Can you work these out from the model? Positions are in its coordinate system, mm. A direction names the side the tool comes from. Coordinates: 2 decimals unless noted, no trailing zeros. Order: outer loops, then holes, each group sorted by start corner. A loop starts at its lowest first (then second) coordinate and runs counter-clockwise, first axis right, second up. Notation, with made-up numbers: (27, 44) -> (77, 44) arc R9 ccw to (77, 49) -> close; hole circle Ø5 at (-36, -11.5). An arc over 180 degrees is marked (long way). Answer as a JSON object with one key per item and string values. Group by question number.
(1) I want a section at B-B, the plane z = 0. List the corners of the cut face in (x, y) for me.
(2) I need wall thicknesses on line 1 (Y direction, x = 1.5, z = -1.75); line 2 (Y direction, x = 1.5, z = 2.75); line 3 (X direction, y = 4.5, z = 0). Which ranges of each line are inside material? Lowest first, please.
(3) Which directions (+Z, -Z, +X, -X, +Y, -Y) give clear straight access to the entire face, cutting with the end or side of a thin tool? Please do faces 4 (the flat face through (0, 0, 0)), 5 (the cylindrical face through (2.024, 23.493, 1.29)), 6 (the flat face through (-2, 22, -1)).
(4) I want a section at D-D, the plane z = 3. List the corners of the cut face in (x, y) for me.
(5) I want a section at A-A, the plane x = 0. List the corners of the cut face in (y, z) for me, plus the area to 3 significant figures.
(6) If we mould it in two halves opening along Y, with no side actions, what happens to faces 1 (the cylindrical face through (-1, 22.49, -1.31)), 2 (the flat face through (0, 24, 0)), 3 (the cylindrical face through (-3.417, 0.493, -0.759))? For each: pulls with the +Y half, pulls with the -Y half, needs draft (parallel to the pull), parting line crosses it, or undercut.
(7) For pin 1 (3 mm diameter, centred on x = 1.5, y = 9, fed in from -Z); pin 2 (2 mm diameter, centred on y = 5.5, z = -3, fed in from +X); pin 3 (1 mm diameter, centred on y = 4.5, z = -2, fed in from +X), each with a flat end and sliding along its axis, tell me the tip position at first contact or that it passes through.
(8) I want a section at C-C, the plane y = 19.75. List the corners of the cut face in (x, z) for me.
from build123d import *

# Parameters (mm, degrees)
CROQUIS1_R              = 3.5
CROQUIS1_R_2            = 2.4
SALIENTE_EXTRUIR1_DEPTH = 1
CROQUIS1_2_R            = 2.4
SALIENTE_EXTRUIR2_DEPTH = 24
CORTAR_EXTRUIR1_START   = -2
CROQUIS2_R              = 2.4
CROQUIS2_R_2            = 1.65
CORTAR_EXTRUIR1_DEPTH   = 1


with BuildPart() as part:
    # Croquis1 → Saliente-Extruir1 (new body)
    with BuildSketch(Plane(origin=(0, 0, 0), x_dir=(1, 0, 0), z_dir=(0, 1, 0))):
        with Locations(Location((0, 0, 0), (0, 0, 270))):
            Circle(CROQUIS1_R)
        with Locations(Location((0, 0, 0), (0, 0, 270))):
            Circle(CROQUIS1_R_2, mode=Mode.SUBTRACT)
    extrude(amount=SALIENTE_EXTRUIR1_DEPTH)

    # Croquis1_2 → Saliente-Extruir2 (add)
    with BuildSketch(Plane(origin=(0, 0, 0), x_dir=(1, 0, 0), z_dir=(0, 1, 0))):
        with Locations(Location((0, 0, 0), (0, 0, 270))):
            Circle(CROQUIS1_2_R)
    extrude(amount=SALIENTE_EXTRUIR2_DEPTH)

    # Croquis2 → Cortar-Extruir1 (cut)
    with BuildSketch(Plane(origin=(0, 24, 0), x_dir=(1, 0, 0), z_dir=(0, 1, 0)).offset(CORTAR_EXTRUIR1_START)):
        with Locations(Location((0, 0, 0), (0, 0, 270))):
            Circle(CROQUIS2_R)
        with Locations(Location((0, 0, 0), (0, 0, 270))):
            Circle(CROQUIS2_R_2, mode=Mode.SUBTRACT)
    extrude(amount=CORTAR_EXTRUIR1_DEPTH, mode=Mode.SUBTRACT)


solid = part.part
Computed values:
{
 "1": {"outline": "(-3.5, 0) -> (3.5, 0) -> (3.5, 1) -> (2.4, 1) -> (2.4, 22) -> (1.65, 22) -> (1.65, 23) -> (2.4, 23) -> (2.4, 24) -> (-2.4, 24) -> (-2.4, 23) -> (-1.65, 23) -> (-1.65, 22) -> (-2.4, 22) -> (-2.4, 1) -> (-3.5, 1) -> close"},
 "2": {"line 1": "y = 0 to 22, 23 to 24", "line 2": "y = 0 to 1", "line 3": "x = -2.4 to 2.4"},
 "3": {"face 4": "+Z, -Z, +X, -X, -Y", "face 5": "+Y", "face 6": "none"},
 "4": {"outline": "(-1.8, 0) -> (1.8, 0) -> (1.8, 1) -> (-1.8, 1) -> close"},
 "5": {"outline": "(0, -3.5) -> (1, -3.5) -> (1, -2.4) -> (22, -2.4) -> (22, -1.65) -> (23, -1.65) -> (23, -2.4) -> (24, -2.4) -> (24, 2.4) -> (23, 2.4) -> (23, 1.65) -> (22, 1.65) -> (22, 2.4) -> (1, 2.4) -> (1, 3.5) -> (0, 3.5) -> close", "area": "116 mm2"},
 "6": {"face 1": "undercut", "face 2": "pulls with the +Y half", "face 3": "needs draft"},
 "7": {"pin 1": "stops at z = -2.4", "pin 2": "stops at x = 1.33", "pin 3": "stops at x = 1.87"},
 "8": {"outline": "circle Ø4.8 at (0, 0)"}
}
